from build123d import *

# Parameters (mm, degrees)
ESQUISSE1_R                  = 2.5
BOSS_EXTRU_1_DEPTH           = 10
ENL_V_MAT_EXTRU_1_DEPTH      = 24.086792761
ENL_V_MAT_EXTRU_1_DEPTH_BACK = 24.086792761
ESQUISSE2_R                  = 2.05


with BuildPart() as part:
    # Esquisse1 → Boss.-Extru.1 (new body)
    with BuildSketch(Plane(origin=(0, 0, 0), x_dir=(0, 0, -1), z_dir=(1, 0, 0))):
        with BuildLine():
            Line((17, 0), (-17, 0))
            Line((-17, 0), (-17, 5))
            Line((-17, 5), (-7, 5))
            Line((-7, 5), (-7, 10))
            ThreePointArc((-7, 10), (0, 17), (7, 10))
            Line((7, 10), (7, 5))
            Line((7, 5), (17, 5))
            Line((17, 5), (17, 0))
        make_face()
        with Locations(Location((0, 10, 0), (0, 0, 180))):
            Circle(ESQUISSE1_R, mode=Mode.SUBTRACT)
    extrude(amount=BOSS_EXTRU_1_DEPTH)

    # Esquisse2 → Enlèv. mat.-Extru.1 (cut, two sides: drawn at the far end of the back side and taken through both)
    with BuildSketch(Plane(origin=(0, 5, 0), x_dir=(1, 0, 0), z_dir=(0, 1, 0)).offset(-ENL_V_MAT_EXTRU_1_DEPTH_BACK)):
        with Locations(Location((5, 12, 0), (0, 0, 270))):
            Circle(ESQUISSE2_R)
        with Locations(Location((5, -12, 0), (0, 0, 270))):
            Circle(ESQUISSE2_R)
    extrude(amount=ENL_V_MAT_EXTRU_1_DEPTH + ENL_V_MAT_EXTRU_1_DEPTH_BACK, mode=Mode.SUBTRACT)


solid = part.part
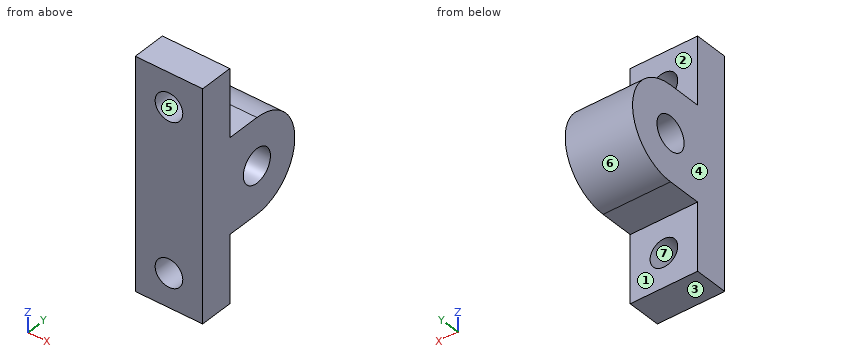
Input: part model. Units: mm. Frame: model coordinates. Face numbers are marked on the shaded views. A direction names the side the tool comes from. Coordinates: 2 decimals unless noted, no trailing zeros. Loops run counter-clockwise (first coordinate to the right, second up) from the corner with the lowest first, then second, coordinate; pieces in that order, holes last. Notation, with made-up numbers: (68, 71.5) -> (84, 71.5) arc R14 ccw to (84, 95.5) -> close; hole circle Ø6 at (44, 56.5). An arc over 180 degrees is marked (long way). Write item = value, one per line. Start each with the question number.
Item 1: Cut plane D-D, the plane x = 7.5. Return loops of the section in (y, z), plus the area to 3 significant figures.
Item 2: Reachability of the marked faces 1, 2 and 3 from +Z, -Z, +X, -X, +Y, -Y: full face, straight path, thin tool, end or side. Return the list, or none.
Item 3: Cut plane A-A, the plane x = 5. Return loops of the section in (y, z), plus the area to 3 significant figures.
Item 4: Cut plane C-C, the plane y = 2. Return loops of the section in (x, z).
Item 5: Cut plane B-B, the plane z = 0. Return loops of the section in (x, y), plus the area to 3 significant figures.
Item 6: Material intervals for line 1 (Z direction, x = 5, y = 1.8); line 2 (Z direction, x = 6, y = 10); line 3 (X direction, y = 1.6, z = 12), sorted ascending.
Item 7: First-contact query: P1, Ø1.5, axis at x = 6.5, z = -3.5, coming from the +Y side; P2, Ø3.5, axis at x = 5, z = 12, coming from the -Y side; P3, Ø4, axis at x = 6, y = 6.5, coming from the +Z side; P4, Ø5, axis at x = 5, z = 11, coming from the +Y side. Flat tips, straight axial feed; report the tip coordinate or a pass-through.
Item 8: Mould query, pull axis X, two halves, no side actions, for the marked faces 4, 5, 6 and 7. Classes: pulls with the +X half, pulls with the -X half, needs draft (parallel to the pull), parting line crosses it, or undercut.
Ans:
q1.outline = (0, -17) -> (5, -17) -> (5, -7) -> (10, -7) arc R7 ccw to (10, 7) -> (5, 7) -> (5, 17) -> (0, 17) -> close; hole circle Ø5 at (10, 0)
q1.area = 297 mm²
q2.face_1 = -Z, +X, -X, +Y
q2.face_2 = +Z, +X, -X, +Y
q2.face_3 = -Z, +X, -X, +Y, -Y
q3.outline = (0, -17) -> (5, -17) -> (5, -14.05) -> (0, -14.05) -> close; (0, -9.95) -> (5, -9.95) -> (5, -7) -> (10, -7) arc R7 ccw to (10, 7) -> (5, 7) -> (5, 9.95) -> (0, 9.95) -> close; (0, 14.05) -> (5, 14.05) -> (5, 17) -> (0, 17) -> close; hole circle Ø5 at (10, 0)
q3.area = 256 mm²
q4.outline = (0, -17) -> (10, -17) -> (10, 17) -> (0, 17) -> close; hole circle Ø4.1 at (5, -12); hole circle Ø4.1 at (5, 12)
q5.outline = (0, 0) -> (10, 0) -> (10, 7.5) -> (0, 7.5) -> close; (0, 12.5) -> (10, 12.5) -> (10, 17) -> (0, 17) -> close
q5.area = 120 mm²
q6.line_1 = -17 to -14.05, -9.95 to 9.95, 14.05 to 17
q6.line_2 = -7 to -2.5, 2.5 to 7
q6.line_3 = 0 to 2.95, 7.05 to 10
q7.P1 = 16.44
q7.P2 = through
q7.P3 = 17
q7.P4 = 5
q8.face_4 = pulls with the -X half
q8.face_5 = undercut
q8.face_6 = needs draft
q8.face_7 = undercut
